Build history of the part. All positions in model axes, mm. Face numbers are marked on the shaded views. A direction names the side the tool comes from. Round coordinates to 2 decimals unless told otherwise and drop trailing zeros. Write each loop counter-clockwise with the first axis right and the second up, starting at its lowest first coordinate (ties: lowest second). Pieces come first, ordered by that corner, then holes.
Item 1: Band-saw the part on A-A, the plane x = -142. Write the cut outline in (y, z) (3 decimals).
Item 2: Band-saw the part on C-C, the plane z = 5. Write the cut outline in (x, y), then the cut area to 3 significant figures.
Item 3: Band-saw the part on B-B, the plane y = 3. Write the cut outline in (x, z) (3 decimals), then the cut area to 3 significant figures.
Item 4: Mould opens along Z. For the marked faces 1, 2 and 3 say: +Z half, -Z half, draft (parallel to the pull), parting line (faces both ways), or undercut.
Item 5: 3-axis set-ups, long thin cutter, end or side, ignore diameter. For the marked faces 4, 5 and 6: which of +Z, -Z, +X, -X, +Y, -Y reach the whole face in a straight line?
Item 6: Band-saw the part on D-D, the plane z = 2.75. Write the cut outline in (x, y), then the cut area to 3 significant figures.
Item 7: Drop flat-ended pins along their axis: pin 1 Ø3 at (x, z) = (-145, 2.5) entering from -Y; pin 2 Ø0.9 at (x, z) = (-145, 4.5) entering from +Y; pin 3 Ø0.9 at (x, z) = (-145.5, 5) entering from -Y. Give the stop position or say it passes through.
Item 8: Wall check: probe 1 along Z at (x, y) = (-149, 2.5); probe 2 along Z at (x, y) = (-150.5, 2.25); probe 3 along Y at (x, z) = (-144, 5). Give the ranges that are in metal, low to high.
```python
from build123d import *

# Parameters (mm, degrees)
SKETCH013_W      = 8.5
SKETCH013_H      = 3.76
EXTRUDE013_DEPTH = 3.54
SKETCH014_W      = 5
SKETCH014_H      = 1.5
EXTRUDE014_DEPTH = 2.97
SKETCH012_W      = 16.69
SKETCH012_H      = 12.65
EXTRUDE012_DEPTH = 1.66


with BuildPart() as extrude_switch_house:
    # Sketch013 → Extrude013 (new body)
    with BuildSketch(Plane.XY):
        with Locations((4.25, 1.88)):
            Rectangle(SKETCH013_W, SKETCH013_H)
    extrude(amount=EXTRUDE013_DEPTH)


with BuildPart() as extrude_switch:
    # Sketch014 → Extrude014 (new body)
    with BuildSketch(Plane.XY):
        with Locations((4.25, 1.88)):
            Rectangle(SKETCH014_W, SKETCH014_H)
    extrude(amount=EXTRUDE014_DEPTH)


with BuildPart() as extrude_switch_1:
    # Extrude014 placement: moved
    add(extrude_switch.part.moved(Location((0, 0, 3.54))))


with BuildPart() as fusion_switch:
    # Sketch012 → Extrude012 (new body)
    with BuildSketch(Plane(origin=(4, 2, 0), x_dir=(1, 0, 0), z_dir=(0, 0, 1))):
        Rectangle(SKETCH012_W, SKETCH012_H)
    extrude(amount=-EXTRUDE012_DEPTH)

    # Fusion004: union Extrude_Switch_house, Extrude_Switch_
    add(extrude_switch_house.part)
    add(extrude_switch_1.part)


with BuildPart() as fusion_switch_1:
    # Fusion004 placement: moved
    add(fusion_switch.part.moved(Location((-150, 0, 0))))


solid = fusion_switch_1.part
```
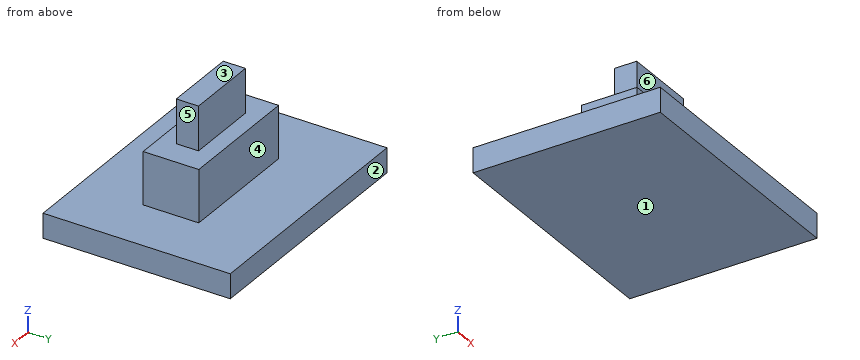
Results:
1. outline: (-4.325, -1.66) - (8.325, -1.66) - (8.325, 0) - (3.76, 0) - (3.76, 3.54) - (0, 3.54) - (0, 0) - (-4.325, 0) - close
2. outline: (-148.25, 1.13) - (-143.25, 1.13) - (-143.25, 2.63) - (-148.25, 2.63) - close
2. area: 7.50 mm2
3. outline: (-154.345, -1.66) - (-137.655, -1.66) - (-137.655, 0) - (-141.5, 0) - (-141.5, 3.54) - (-150, 3.54) - (-150, 0) - (-154.345, 0) - close
3. area: 57.8 mm2
4. face 1: -Z half
4. face 2: draft
4. face 3: +Z half
5. face 4: +Z, +X, -X, +Y
5. face 5: +Z, +X, +Y, -Y
5. face 6: +Z, +X, -X, -Y
6. outline: (-150, 0) - (-141.5, 0) - (-141.5, 3.76) - (-150, 3.76) - close
6. area: 32.0 mm2
7. pin 1: stops at y = 0
7. pin 2: stops at y = 2.63
7. pin 3: stops at y = 1.13
8. probe 1: z = -1.66 to 3.54
8. probe 2: z = -1.66 to 0
8. probe 3: y = 1.13 to 2.63
